Work out the finished part from the listing and answer in its coordinate system (mm). A direction names the side the tool comes from. Round coordinates to 2 decimals unless told otherwise and drop trailing zeros. Write each loop counter-clockwise with the first axis right and the second up, starting at its lowest first coordinate (ties: lowest second). Pieces come first, ordered by that corner, then holes. Notation, with made-up numbers: (84.25, -26.75) -> (96.25, -26.75) arc R26 ccw to (96.25, -4.75) -> close; hole circle Ø4 at (-8, 0). An arc over 180 degrees is marked (long way). One line per item, written item: value.
```python
from build123d import *

# Parameters (mm, degrees)
BOSS_EXTRUDE1_DEPTH     = 9.525
CUT_EXTRUDE2_DEPTH      = 139.148989433
CUT_EXTRUDE2_DEPTH_BACK = 139.148989433
SKETCH6_R               = 2.286
SKETCH7_R               = 2.286
CUT_EXTRUDE3_DEPTH      = 12.7
FILLET3_R               = 76.2
FILLET4_R               = 1.5875
FILLET5_R               = 4.7625
CUT_EXTRUDE4_DEPTH      = 129.978879691
CUT_EXTRUDE4_DEPTH_BACK = 129.978879691
FILLET6_R               = 1.5875


with BuildPart() as part:
    # Sketch1 → Boss-Extrude1 (new body)
    with BuildSketch(Plane(origin=(0, 0, 0), x_dir=(1, 0, 0), z_dir=(0, 1, 0))):
        Polygon((-28.575, 4.7625), (-28.575, -4.7625), (-6.35, -115.8875), (-6.35, -125.4125), (6.35, -125.4125), (6.35, -115.8875), (28.575, -4.7625), (28.575, 4.7625), align=None)
    extrude(amount=BOSS_EXTRUDE1_DEPTH)

    # Sketch6 → Cut-Extrude2 (cut, two sides: drawn at the far end of the back side and taken through both)
    with BuildSketch(Plane.ZY.offset(28.575).offset(-CUT_EXTRUDE2_DEPTH_BACK)):
        with Locations((0, 4.7625)):
            Circle(SKETCH6_R)
    extrude(amount=CUT_EXTRUDE2_DEPTH + CUT_EXTRUDE2_DEPTH_BACK, mode=Mode.SUBTRACT)

    # Sketch7 → Cut-Extrude3 (cut)
    with BuildSketch(Plane.XY.offset(125.4125)):
        with Locations((0, 4.7625)):
            Circle(SKETCH7_R)
    extrude(amount=-CUT_EXTRUDE3_DEPTH, mode=Mode.SUBTRACT)

    # Fillet3
    fillet3_edges = [part.edges().sort_by_distance(p)[0] for p in [
        (6.35, 4.7625, 115.8875),
        (-6.35, 4.7625, 115.8875),
    ]]
    fillet(fillet3_edges, radius=FILLET3_R)

    # Fillet4
    fillet4_edges = [part.edges().sort_by_distance(p)[0] for p in [
        (6.35, 4.7625, 125.4125),
        (-6.35, 4.7625, 125.4125),
    ]]
    fillet(fillet4_edges, radius=FILLET4_R)

    # Fillet5
    fillet5_edges = [part.edges().sort_by_distance(p)[0] for p in [
        (0, 0, -4.7625),
        (0, 9.525, -4.7625),
    ]]
    fillet(fillet5_edges, radius=FILLET5_R - 0.0001)  # a hair under: the kernel refuses the full size

    # Sketch8 → Cut-Extrude4 (cut, two sides: drawn at the far end of the back side and taken through both)
    with BuildSketch(Plane(origin=(0, 9.525, 0), x_dir=(1, 0, 0), z_dir=(0, 1, 0)).offset(-CUT_EXTRUDE4_DEPTH_BACK)):
        with BuildLine():
            ThreePointArc((-3.159737044, -107.554734345), (-3.120475766, -107.752318634), (-3.081706229, -107.95))
            Line((-3.081706229, -107.95), (3.081706229, -107.95))
            ThreePointArc((3.081706229, -107.95), (3.120475766, -107.752318634), (3.159737044, -107.554734345))
            Line((3.159737044, -107.554734345), (6.573183913, -90.4875))
            Line((6.573183913, -90.4875), (-6.573183913, -90.4875))
            Line((-6.573183913, -90.4875), (-3.159737044, -107.554734345))
        make_face()
        Polygon((0, -64.734965609), (-9.740127938, -74.652779875), (-7.208183913, -87.3125), (7.208183913, -87.3125), (9.740127938, -74.652779875), align=None)
        Polygon((10.493050249, -70.888168322), (14.721754664, -49.744646246), (2.225043776, -62.469331006), align=None)
        Polygon((-2.225043776, -62.469331006), (-14.721754664, -49.744646246), (-10.493050249, -70.888168322), align=None)
        Polygon((13.045786034, -46.919919878), (0, -34.107860525), (-13.045786034, -46.919919878), (0, -60.203696402), align=None)
        Polygon((-2.265634604, -31.882816749), (-22.211903335, -12.29390289), (-15.662709625, -45.03987144), align=None)
        Polygon((20.50004931, -9.525), (-20.50004931, -9.525), (0, -29.657772974), align=None)
        Polygon((15.662709625, -45.03987144), (22.211903335, -12.29390289), (2.265634604, -31.882816749), align=None)
    extrude(amount=CUT_EXTRUDE4_DEPTH + CUT_EXTRUDE4_DEPTH_BACK, mode=Mode.SUBTRACT)

    # Fillet6
    fillet6_edges = [part.edges().sort_by_distance(p)[0] for p in [
        (3.081706229, 4.7625, 107.95),
        (-3.081706229, 4.7625, 107.95),
        (-6.573183913, 4.7625, 90.4875),
        (6.573183913, 4.7625, 90.4875),
        (-15.662709625, 4.7625, 45.03987144),
        (-22.211903335, 4.7625, 12.29390289),
        (-2.265634604, 4.7625, 31.882816749),
        (2.265634604, 4.7625, 31.882816749),
        (22.211903335, 4.7625, 12.29390289),
        (15.662709625, 4.7625, 45.03987144),
        (10.493050249, 4.7625, 70.888168322),
        (2.225043776, 4.7625, 62.469331006),
        (14.721754664, 4.7625, 49.744646246),
        (9.740127938, 4.7625, 74.652779875),
        (7.208183913, 4.7625, 87.3125),
        (-7.208183913, 4.7625, 87.3125),
        (-9.740127938, 4.7625, 74.652779875),
        (13.045786034, 4.7625, 46.919919878),
        (0, 4.7625, 60.203696402),
        (-13.045786034, 4.7625, 46.919919878),
        (0, 4.7625, 34.107860525),
        (-2.225043776, 4.7625, 62.469331006),
        (-10.493050249, 4.7625, 70.888168322),
        (-14.721754664, 4.7625, 49.744646246),
        (20.50004931, 4.7625, 9.525),
        (0, 4.7625, 29.657772974),
        (-20.50004931, 4.7625, 9.525),
        (0, 4.7625, 64.734965609),
    ]]
    fillet(fillet6_edges, radius=FILLET6_R)


solid = part.part
```
(1) For a pull along Y with two mould halves and no side action, classify faces 1 (the face through (0, 5, 112.712)), 2 (the face through (12.3, 0, 47.9)), 3 (the face through (-10, 4.83, 69.15)) as pulls with the +Y half, pulls with the -Y half, needs draft (parallel to the pull), parting line crosses it, or undercut.
Reported:
face 1: undercut
face 2: pulls with the -Y half
face 3: needs draft
(2) Consider probe 1 along Y at (x, z) = (0, 119) (1 decimal); probe 2 along X at (y, z) = (7, 18); probe 3 along X at (y, z) = (4.75, 55). Determine where each line is inside the solid, lowest interval first.
Reported:
probe 1: y = 0 to 2.5, 7 to 9.5
probe 2: x = -25.93 to -21.07, -16.4 to -11.87, 11.87 to 16.4, 21.07 to 25.93
probe 3: x = -18.53 to -13.67, -9.56 to -5.11, 5.11 to 9.56, 13.67 to 18.53
(3) Find section C-C on z = 117. Give the vertices of the cut face in (x, y) (1 decimal).
Reported:
outline: (-6.6, 0) -> (6.6, 0) -> (6.6, 9.5) -> (-6.6, 9.5) -> close; hole circle Ø4.6 at (0, 4.8)
(4) Flat-ended cylindrical pins translate along their axes: pin 1 Ø3 at (y, z) = (3, 14) entering from +X; pin 2 Ø5 at (y, z) = (7.5, 37) entering from -X; pin 3 Ø1.8 at (x, y) = (1, 3) entering from -Z. Find the tip coordinate at first contact, or state that the pin passes through.
Reported:
pin 1: stops at x = 27.03
pin 2: stops at x = -22.63
pin 3: stops at z = -4.68
(5) A tool of negligible diameter and unlimited length cuts with its end or side. For faces 4 (the face through (6.71, 4.83, 116.03)), 5 (the face through (9.305, 4.696, 20.519)), from which of +Z, -Z, +X, -X, +Y, -Y can it reach the whole face along a straight path? Write none if from no direction.
Reported:
face 4: +Z, +X, +Y, -Y
face 5: +Y, -Y
(6) Find section A-A on z = 22. Give the vertices of the cut face in (x, y) (1 decimal), plus the area to 3 significant figures.
Reported:
outline: (-25.1, 0) -> (-20.3, 0) -> (-20.3, 9.5) -> (-25.1, 9.5) -> close; (-12.3, 0) -> (-7.8, 0) -> (-7.8, 9.5) -> (-12.3, 9.5) -> close; (7.8, 0) -> (12.3, 0) -> (12.3, 9.5) -> (7.8, 9.5) -> close; (20.3, 0) -> (25.1, 0) -> (25.1, 9.5) -> (20.3, 9.5) -> close
area: 179 mm2
